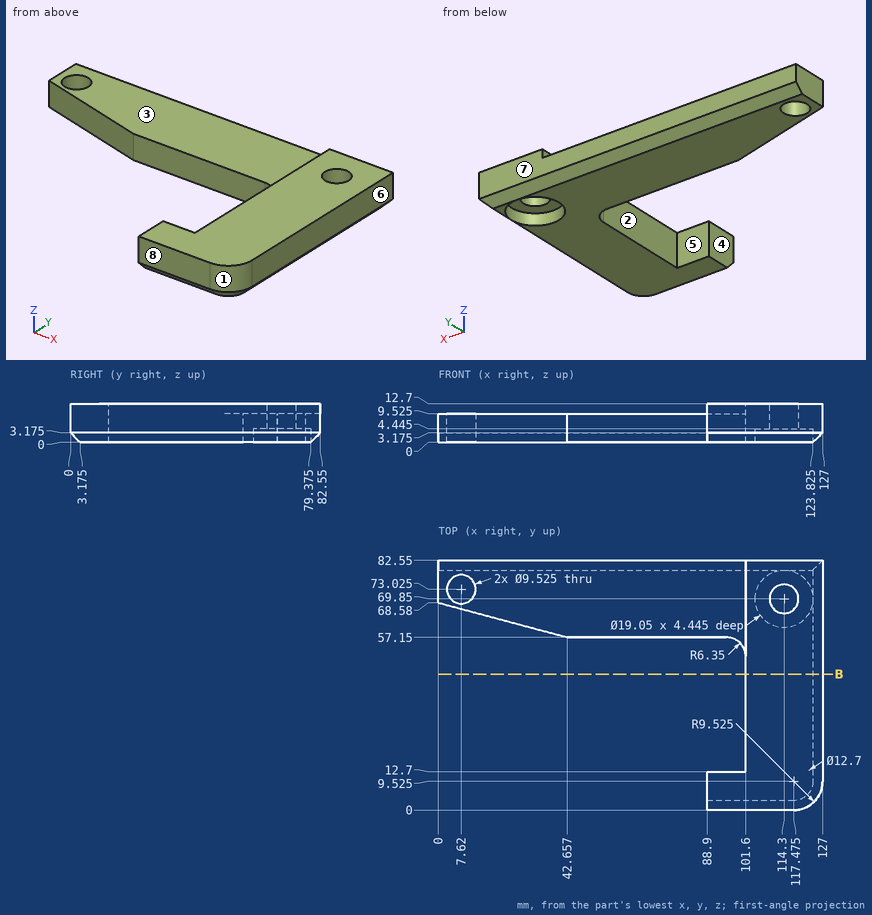
Here's the drawing with two shaded views (mm, measured from the low corner). I have some questions. A direction names the side the tool comes from. Round coordinates to 2 decimals unless told otherwise and drop trailing zeros. Loops run counter-clockwise (first coordinate to the right, second up) from the corner with the lowest first, then second, coordinate; pieces in that order, holes last. Notation, with made-up numbers: M 34,-3.5 L 72,-3.5 A21 ccw 72,26.5 Z; hole C -8,48.5 d11. An arc over 180 degrees is marked long. Answer as CSV lines item,"result".
1) We'd pull the mould along Y, two halves only. Please class the marked faces 5, 6, 7 and 8: released by +Y, released by -Y, zero draft, split by the parting line, or undercut.
From the geometry:
face 5,"undercut"
face 6,"zero draft"
face 7,"released by +Y"
face 8,"released by -Y"
2) Imagine slicing it at B-B on y = 45. List the corners of the cut face in (x, z) for me (1 decimal).
From the geometry:
outline,"M 101.6,0 L 123.8,0 L 127,3.2 L 127,12.7 L 101.6,12.7 Z"
3) For pin 1 Ø5 at (x, z) = (82, 3) entering from -Y; pin 2 Ø12.5 at (x, y) = (114.3, 69.85) entering from -Z (3 decimals); pin 3 Ø5 at (y, z) = (52, 10) entering from -X, each with a flat end and sliding along its axis, tell me the tip position at first contact or that it passes through.
From the geometry:
pin 1,"y = 57.15"
pin 2,"z = 4.445"
pin 3,"x = 100.44"
4) Which directions (+Z, -Z, +X, -X, +Y, -Y) give clear straight access to the entire face, cutting with the end or side of a thin tool? Please do the marked faces 1, 2, 3 and 4.
From the geometry:
face 1,"+Z, -Z, +X, -Y"
face 2,"+Z, -X"
face 3,"+Z, -X, +Y"
face 4,"+Z, -Z, -X, -Y"
5) If I drill on probe 1 along X at (y, z) = (72.5, 4.75) (1 decimal); probe 2 along Y at (x, z) = (114.3, 8); probe 3 along X at (y, z) = (23.5, 9.25), over which ranges is the centre line in solid material (lowest first)?
From the geometry:
probe 1,"0 to 2.9, 12.4 to 110.3, 118.3 to 127"
probe 2,"0 to 65.09, 74.61 to 82.55"
probe 3,"101.6 to 127"
